```python
from build123d import *

# Parameters (mm, degrees)
SKETCH1_W           = 21.293186277
SKETCH1_H           = 6.556248908
SKETCH1_R           = 2.06
SKETCH1_R_2         = 2.04
SKETCH1_R_3         = 2.05
BOSS_EXTRUDE1_DEPTH = 10
FILLET1_R           = 2


with BuildPart() as part:
    # Sketch1 → Boss-Extrude1 (new body)
    with BuildSketch(Plane(origin=(0, 0, 0), x_dir=(1, 0, 0), z_dir=(0, 1, 0))):
        with Locations((10.646593139, 3.278124454)):
            Rectangle(SKETCH1_W, SKETCH1_H)
        with Locations(Location((17.959518774, 3.152151811, 0), (0, 0, 270))):
            Circle(SKETCH1_R, mode=Mode.SUBTRACT)
        with Locations(Location((3.502477391, 3.152151811, 0), (0, 0, 270))):
            Circle(SKETCH1_R_2, mode=Mode.SUBTRACT)
        with Locations(Location((10.712545691, 3.152151811, 0), (0, 0, 270))):
            Circle(SKETCH1_R_3, mode=Mode.SUBTRACT)
    extrude(amount=BOSS_EXTRUDE1_DEPTH)

    # Fillet1
    # the kernel refuses this fillet: 2 mm, written as the material it takes off along each edge
    with BuildSketch(Plane(origin=(-5, 10, 0), x_dir=(0, -1, 0), z_dir=(1, 0, 0))) as fillet1_piece_1:
        with BuildLine():
            CenterArc((FILLET1_R, FILLET1_R), FILLET1_R, 180, 90)
            Line((0, FILLET1_R), (0, 0))
            Line((0, 0), (FILLET1_R, 0))
        make_face()
    extrude(amount=31.293186277, mode=Mode.SUBTRACT)
    with BuildSketch(Plane(origin=(0, 10, -11.556248908), x_dir=(0, -1, 0), z_dir=(0, 0, 1))) as fillet1_piece_2:
        with BuildLine():
            CenterArc((FILLET1_R, FILLET1_R), FILLET1_R, 180, 90)
            Line((0, FILLET1_R), (0, 0))
            Line((0, 0), (FILLET1_R, 0))
        make_face()
    extrude(amount=16.556248908, mode=Mode.SUBTRACT)


solid = part.part
```
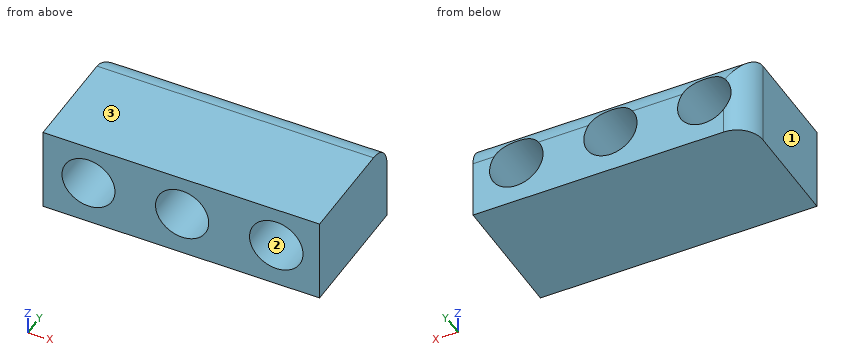
Input: part model. Units: mm. Frame: model coordinates. Face numbers are marked on the shaded views. Give positions to 0.01 mm unless a question says otherwise; leave off trailing zeros. Order: outer loops, then holes, each group sorted by start corner. A loop starts at its lowest first (then second) coordinate and runs counter-clockwise, first axis right, second up.
1. Section A-A on x = 3. Return the cut outline in (y, z) (3 decimals).
Derived:
outline: (0, -6.556) - (10, -6.556) - (10, -5.129) - (0, -5.129) - close; (0, -1.175) - (9.822, -1.175) arc R2 ccw to (8, 0) - (0, 0) - close
2. Section C-C on y = 5.5. Return the cut outline in (x, z).
Derived:
outline: (0, -6.56) - (21.29, -6.56) - (21.29, 0) - (0, 0) - close; hole circle Ø4.08 at (3.5, -3.15); hole circle Ø4.1 at (10.71, -3.15); hole circle Ø4.12 at (17.96, -3.15)
3. Mould query, pull axis Z, two halves, no side actions, for the marked faces 1, 2 and 3. Classes: released by +Z, released by -Z, zero draft, split by the parting line, or undercut.
Derived:
face 1: zero draft
face 2: undercut
face 3: released by +Z
4. Material intervals for L1, parallel to X at y = 5.25, z = -3; L2, parallel to X at y = 2, z = -2; L3, parallel to Z at x = 17.75, y = 1.25, sorted ascending.
Derived:
L1: x = 0 to 1.47, 5.54 to 8.67, 12.76 to 15.91, 20.01 to 21.29
L2: x = 0 to 1.82, 5.19 to 9.02, 12.41 to 16.25, 19.67 to 21.29
L3: z = -6.56 to -5.2, -1.1 to 0
5. Section B-B on z = -3.5. Return the cut outline in (x, y), and give its area (3 significant figures).
Derived:
outline: (0, 0) - (1.49, 0) - (1.49, 9.93) arc R2 ccw to (0, 8) - close; (5.51, 0) - (8.69, 0) - (8.69, 10) - (5.51, 10) - close; (12.73, 0) - (15.93, 0) - (15.93, 10) - (12.73, 10) - close; (19.99, 0) - (21.29, 0) - (21.29, 10) - (19.99, 10) - close
area: 90.9 mm2
6. Section D-D on z = -1.5. Return the cut outline in (x, y), and give its area (3 significant figures).
Derived:
outline: (0, 0) - (2.31, 0) - (2.31, 9.94) - (1.5, 9.94) arc R2 ccw to (0, 8) - close; (4.7, 0) - (9.5, 0) - (9.5, 9.94) - (4.7, 9.94) - close; (11.93, 0) - (16.73, 0) - (16.73, 9.94) - (11.93, 9.94) - close; (19.19, 0) - (21.29, 0) - (21.29, 9.94) - (19.19, 9.94) - close
area: 138 mm2
